```python
from build123d import *

# Parameters (mm, degrees)
F0_R          = 7.5
F1_DEPTH      = 8
F2_DEPTH      = 5
F2_DEPTH_BACK = 30
F4_DEPTH      = 12.5
F5_DEPTH      = 10
F5_DEPTH_BACK = 25
F7_DEPTH      = 25
F7_DEPTH_BACK = 25


with BuildPart() as f1:
    # F0 (on Right) → F1 (new body)
    with BuildSketch(Plane.YZ):
        with BuildLine():
            ThreePointArc((0, -10), (7.0710678119, -7.0710678119), (10, 0))
            ThreePointArc((10, 0), (-7.0710678119, 7.0710678119), (0, -10))
        make_face()
        Circle(F0_R, mode=Mode.SUBTRACT)
    extrude(amount=F1_DEPTH)

    # F0 (on Right) → F2 (join, two sides)
    with BuildSketch(Plane.YZ) as f2_sk:
        with BuildLine():
            ThreePointArc((0, -10), (7.0710678119, -7.0710678119), (10, 0))
            ThreePointArc((10, 0), (-7.0710678119, 7.0710678119), (0, -10))
        make_face()
        Circle(F0_R, mode=Mode.SUBTRACT)
    extrude(amount=F2_DEPTH)
    extrude(f2_sk.sketch, amount=-F2_DEPTH_BACK)

    # F3 (on Front) → F4 (cut, symmetric)
    with BuildSketch(Plane.XZ):
        Polygon((8, 0), (8, 10), (3.417424305, 10), align=None)
    extrude(amount=F4_DEPTH, both=True, mode=Mode.SUBTRACT)

    # F0 (on Right) → F5 (join, two sides)
    with BuildSketch(Plane.YZ) as f5_sk:
        with BuildLine():
            ThreePointArc((13.5738675599, -10.038333654), (10.9801111189, -5.3064134392), (10, 0))
            ThreePointArc((10, 0), (7.0710678119, -7.0710678119), (0, -10))
            ThreePointArc((0, -10), (5.3064134392, -10.9801111189), (10.038333654, -13.5738675599))
            Line((10.038333654, -13.5738675599), (27.0088964024, -30.5444303084))
            Line((27.0088964024, -30.5444303084), (30.5444303084, -27.0088964024))
            Line((30.5444303084, -27.0088964024), (13.5738675599, -10.038333654))
        make_face()
    extrude(amount=-F5_DEPTH)
    extrude(f5_sk.sketch, amount=F5_DEPTH_BACK)

    # F6 (on face) → F7 (cut, two sides)
    with BuildSketch(Plane(origin=(0, 1.767766953, 1.767766953), x_dir=(1, 0, 0), z_dir=(0, 0.7071067812, 0.7071067812))) as f7_sk:
        with BuildLine():
            ThreePointArc((-10, 10), (-7.1369616608, 13.3518740219), (-4.2652819266, 16.6963475971))
            Line((-4.2652819266, 16.696347597), (-10, 16.696347597))
            Line((-10, 16.696347597), (-10, 10))
        make_face()
        with BuildLine():
            ThreePointArc((-4.2652819266, 16.6963475971), (6.2060505049, 28.7455446955), (16.7895406485, 40.696347597))
            Line((16.7895406485, 40.696347597), (-10, 40.696347597))
            Line((-10, 40.696347597), (-10, 16.696347597))
            Line((-10, 16.696347597), (-4.2652819266, 16.696347597))
        make_face()
        with BuildLine():
            Line((25, 16.696347597), (25, 40.696347597))
            ThreePointArc((25, 40.696347597), (17.0783625635, 29.2519356675), (11.071357295, 16.696347597))
            Line((11.071357295, 16.696347597), (25, 16.696347597))
        make_face()
        with BuildLine():
            Line((25, 16.696347597), (11.071357295, 16.696347597))
            ThreePointArc((11.071357295, 16.696347597), (9.396655894, 11.9280688615), (8, 7.0710678119))
            Line((8, 7.0710678119), (25, 7.0189046673))
            Line((25, 7.0189046673), (25, 16.696347597))
        make_face()
    extrude(amount=-F7_DEPTH, mode=Mode.SUBTRACT)
    extrude(f7_sk.sketch, amount=F7_DEPTH_BACK, mode=Mode.SUBTRACT)


solid = f1.part
```
Could you check a few things on this model? Use its own coordinates, in mm. A direction names the side the tool comes from. Round coordinates to 2 decimals unless told otherwise and drop trailing zeros. Loops run counter-clockwise (first coordinate to the right, second up) from the corner with the lowest first, then second, coordinate; pieces in that order, holes last.
Q1. I want a section at C-C (x = -14). Write out the boundary of the cut face in (y, z), and give its area (3 significant figures).
Q2. Please list where these lines run through material, in increasing order: L1, parallel to Z at x = -17.5, y = 0; L2, parallel to Z at x = -20, y = -4.
Q3. I want a section at B-B (z = 2). Write out the boundary of the cut face in (x, y).
Q4. I want a section at A-A (x = -7). Write out the boundary of the cut face in (y, z).
Q5. On a 3-axis mill with a long thin cutter (end or side, diameter ignored), from which of +Z, -Z, +X, -X, +Y, -Y can I reach the whole of each face in a straight line? I mean faces 1 (the cylindrical face through (8.31, 7.15, -6.99)), 2 (the flat face through (-10, 9.53, -3.52)), 3 (the flat face through (4.66, -2.36, 7.29)). Say none if no direction works.
Q6. For P1, Ø1.5, axis at x = 12, y = 16, coming from the -Z side; P2, Ø5, axis at y = 5, z = -4, coming from the +X side; P3, Ø6, axis at y = 1, z = -2.5, coming from the -X side; P4, Ø12, axis at x = -16, z = -9.5, coming from the -Y side, each with a flat end and sliding along its axis, tell me the tip position at first contact or that it passes through.
Answer below:
1. outline: circle Ø20 at (0, 0); hole circle Ø15 at (0, 0)
1. area: 137 mm2
2. L1: z = -10 to -7.5, 7.5 to 10
2. L2: z = -9.17 to -6.34, 6.34 to 9.17
3. outline: (-30, -9.8) - (7.08, -9.8) - (7.08, -7.23) - (-30, -7.23) - close; (-30, 7.23) - (7.08, 7.23) - (7.08, 9.8) - (-30, 9.8) - close
4. outline: (0, -10) arc R17 cw to (7.28, -11.83) - (11.83, -7.28) arc R17 cw to (10, 0) arc R10 ccw (long way) to start; hole circle Ø15 at (0, 0)
5. face 1: +Z, +X, -Y
5. face 2: -Z, -X, +Y
5. face 3: +Z, +X, +Y, -Y
6. P1: stops at z = -20.29
6. P2: stops at x = 8
6. P3: passes through
6. P4: stops at y = -9.37
